from build123d import *

# Parameters (mm, degrees)
SKETCH2_R          = 10
CUT_EXTRUDE1_DEPTH = 46
SKETCH3_R          = 5
CUT_EXTRUDE2_DEPTH = 29


with BuildPart() as part:
    # Sketch1 → Revolve1 (revolve)
    with BuildSketch(Plane(origin=(0, 0, 0), x_dir=(0, 1, 0), z_dir=(0, 0, 1))):
        Polygon((0, 0), (35, 0), (40, 0), (40, 16), (23, 18), (23, 35), (35, 38), (35, 43), (0, 43), (0, 38), (12, 35), (12, 18), (-5, 16), (-5, 0), align=None)
    revolve(axis=Axis((0, 0, 0), (0, 1, 0)))

    # Sketch2 → Cut-Extrude1 (cut, through all)
    with BuildSketch(Plane.XZ.offset(5)):
        Circle(SKETCH2_R)
    extrude(amount=-CUT_EXTRUDE1_DEPTH, mode=Mode.SUBTRACT)

    # Sketch3 → Cut-Extrude2 (cut, through all)
    with BuildSketch(Plane(origin=(0, 23, 0), x_dir=(-1, 0, 0), z_dir=(0, 1, 0))):
        with Locations((0, 26.5)):
            Circle(SKETCH3_R)
        with Locations((26.5, 0)):
            Circle(SKETCH3_R)
        with Locations((0, -26.5)):
            Circle(SKETCH3_R)
        with Locations((-26.5, 0)):
            Circle(SKETCH3_R)
    extrude(amount=-CUT_EXTRUDE2_DEPTH, mode=Mode.SUBTRACT)


solid = part.part
Design review of the part built by this model. Coordinates are the model's own, in mm. A direction names the side the tool comes from. Coordinates: 2 decimals unless noted, no trailing zeros. Write each loop counter-clockwise with the first axis right and the second up, starting at its lowest first coordinate (ties: lowest second). Pieces come first, ordered by that corner, then holes. Notation, with made-up numbers: (80.25, 42) - (107.25, 42) arc R30 cw to (107.25, 81) - close; hole circle Ø7 at (-16, 43.5). An arc over 180 degrees is marked (long way). Use one line per item in the form item = value.
Q1. For probe 1 along Z at (x, y) = (0, 19.5); probe 2 along Z at (x, y) = (-3.5, 15); probe 3 along Z at (x, y) = (11, 25.5), list the stretches that pass through material, from the lowest coordinate up.
Taken from the geometry:
probe_1 = -43 to -31.5, -21.5 to -10, 10 to 21.5, 31.5 to 43
probe_2 = -42.86 to -30.07, -22.93 to -9.37, 9.37 to 22.93, 30.07 to 42.86
probe_3 = -41.57 to -33.88, -13.87 to 13.87, 33.88 to 41.57
Q2. Machinability: for faces 5 (the cylindrical face through (-2.17, 17.18, -9.76)), 6 (the flat face through (16, 35, -35)), 7 (the flat face through (-15, 12, -15)), which of the approach directions +Z, -Z, +X, -X, +Y, -Y give a long, thin tool a straight path to every point of the face, cutting with its end or side? Answer none if there is none.
Taken from the geometry:
face_5 = +Y, -Y
face_6 = +Y
face_7 = -Y
Q3. Consider section A-A (z = 0). Count the separate pieces of the cut face and the enclosed holes in it, plus the area to 3 significant figures.
Taken from the geometry:
separate_pieces = 4
enclosed_holes = 0
area = 1,290 mm^2
Q4. Consider section D-D (y = 30). Write out the cut boundary in (x, z), plus the area to 3 significant figures.
Taken from the geometry:
outline = circle Ø86 at (0, 0); circle Ø34.35 at (0, 0); hole circle Ø73.5 at (0, 0); hole circle Ø20 at (0, 0)
area = 2,180 mm^2
Q5. Consider section B-B (y = 6). Write out the cut boundary in (x, z), plus the area to 3 significant figures.
Taken from the geometry:
outline = circle Ø86 at (0, 0); circle Ø34.59 at (0, 0); hole circle Ø73 at (0, 0); hole circle Ø20 at (0, 0)
area = 2,250 mm^2
Q6. The part is to be moulded in two halves that separate along X. For faces 1 (the flat face through (15, 23, -15)), 2 (the cylindrical face through (5.598, 17.255, 42.634)), 3 (the flat face through (0.2, -5, -10.4)), 4 (the cylindrical face through (1.08, 17.58, 21.62)), say which applies: +X half, -X half, draft (parallel to the pull), parting line (faces both ways), or undercut.
Taken from the geometry:
face_1 = undercut
face_2 = parting line
face_3 = draft
face_4 = undercut
Q7. Consider section C-C (y = 37). Write out the cut boundary in (x, z), plus the area to 3 significant figures.
Taken from the geometry:
outline = circle Ø32.71 at (0, 0); hole circle Ø20 at (0, 0)
area = 526 mm^2
Q8. Insertion check: pin 1 Ø6 at (y, z) = (5.5, -6) entering from -X; pin 2 Ø12 at (x, z) = (-33.5, 20.5) entering from +Y; pin 3 Ø12 at (y, z) = (11.5, -16) entering from -X. Each pin has a flat end and moves straight along its axis. Give the tip position at first contact, or say it passes through.
Taken from the geometry:
pin_1 = -42.9
pin_2 = 35
pin_3 = -41.82
